from build123d import *

# Parameters (mm, degrees)
CROQUIS1_W              = 51
CROQUIS1_H              = 39
CROQUIS1_W_2            = 47
CROQUIS1_H_2            = 35
SALIENTE_EXTRUIR1_DEPTH = 36
CROQUIS2_W              = 51
CROQUIS2_H              = 39
SALIENTE_EXTRUIR2_DEPTH = 2
CROQUIS3_W              = 5
CROQUIS3_H              = 39
SALIENTE_EXTRUIR3_DEPTH = 2
CROQUIS4_W              = 51
CROQUIS4_H              = 2
CORTAR_EXTRUIR1_DEPTH   = 50.744346412
CROQUIS5_W              = 3
CROQUIS5_H              = 2
SALIENTE_EXTRUIR4_DEPTH = 35
REDONDEO1_R             = 2
CHAFL_N1_SIZE           = 1
CROQUIS6_W              = 35
CROQUIS6_H              = 10
CORTAR_EXTRUIR2_DEPTH   = 66.40068807


with BuildPart() as part:
    # Croquis1 → Saliente-Extruir1 (new body)
    with BuildSketch(Plane(origin=(0, 0, 0), x_dir=(1, 0, 0), z_dir=(0, 1, 0))):
        Rectangle(CROQUIS1_W, CROQUIS1_H)
        Rectangle(CROQUIS1_W_2, CROQUIS1_H_2, mode=Mode.SUBTRACT)
    extrude(amount=SALIENTE_EXTRUIR1_DEPTH)

    # Croquis2 → Saliente-Extruir2 (add)
    with BuildSketch(Plane.XZ):
        Rectangle(CROQUIS2_W, CROQUIS2_H)
    extrude(amount=SALIENTE_EXTRUIR2_DEPTH)

    # Croquis3 → Saliente-Extruir3 (add)
    with BuildSketch(Plane(origin=(0, 36, 0), x_dir=(1, 0, 0), z_dir=(0, 1, 0))):
        with Locations((-23, 0)):
            Rectangle(CROQUIS3_W, CROQUIS3_H)
        with Locations((23, 0)):
            Rectangle(CROQUIS3_W, CROQUIS3_H)
    extrude(amount=-SALIENTE_EXTRUIR3_DEPTH)

    # Croquis4 → Cortar-Extruir1 (cut, through all)
    with BuildSketch(Plane(origin=(0, 36, 0), x_dir=(1, 0, 0), z_dir=(0, 1, 0))):
        with Locations((0, -18.5)):
            Rectangle(CROQUIS4_W, CROQUIS4_H)
    extrude(amount=-CORTAR_EXTRUIR1_DEPTH, mode=Mode.SUBTRACT)

    # Croquis5 → Saliente-Extruir4 (add)
    with BuildSketch(Plane.XY.offset(17.5)):
        with Locations((-22, 30)):
            Rectangle(CROQUIS5_W, CROQUIS5_H)
        with Locations((22, 30)):
            Rectangle(CROQUIS5_W, CROQUIS5_H)
    extrude(amount=-SALIENTE_EXTRUIR4_DEPTH)

    # Redondeo1
    redondeo1_edges = [part.edges().sort_by_distance(p)[0] for p in [
        (-25.5, 36, -1),
        (0, 36, -19.5),
        (25.5, 36, -1),
    ]]
    fillet(redondeo1_edges, radius=REDONDEO1_R - 0.0001)  # a hair under: the kernel refuses the full size

    # Chaflán1
    chafl_n1_edges = [part.edges().sort_by_distance(p)[0] for p in [
        (-22, 31, 17.5),
        (22, 31, 17.5),
        (-22, 34, 17.5),
        (22, 34, 17.5),
    ]]
    chamfer(chafl_n1_edges, length=CHAFL_N1_SIZE)

    # Croquis6 → Cortar-Extruir2 (cut, through all)
    with BuildSketch(Plane(origin=(25.5, 0, 0), x_dir=(0, 0, -1), z_dir=(1, 0, 0))):
        with Locations((0, 3)):
            Rectangle(CROQUIS6_W, CROQUIS6_H)
    extrude(amount=-CORTAR_EXTRUIR2_DEPTH, mode=Mode.SUBTRACT)


solid = part.part
The model under review builds one solid part; all positions refer to its coordinate system, in mm. A direction names the side the tool comes from. Give positions to 0.01 mm unless a question says otherwise; leave off trailing zeros. Write each loop counter-clockwise with the first axis right and the second up, starting at its lowest first coordinate (ties: lowest second). Pieces come first, ordered by that corner, then holes. Notation, with made-up numbers: M -26.75,80 L 6.25,80 A27 ccw 6.25,99 Z; hole C 58,52.25 d5. An arc over 180 degrees is marked long. One line per question, with ' | ' between items. Start each with the question number.
Item 1: For faces 4 (the flat face through (-22, 34, -1)), 5 (the flat face through (-22, 29, 0)), 6 (the flat face through (-20.5, 35, 0)), 7 (the flat face through (-24, 8, 0)), list the 3-axis set-ups (+Z, -Z, +X, -X, +Y, -Y) from which the entire face can be reached by the end or side of a thin tool; tool diameter is ignored.
Item 2: We need section B-B on y = 15.5. Write out the cut boundary in (x, z), plus the area to 3 significant figures.
Item 3: For pin 1 (11.5 mm diameter, centred on x = 12.5, y = 12.5, fed in from +Z); pin 2 (2.5 mm diameter, centred on x = 21.5, z = 1, fed in from -Y); pin 3 (1.6 mm diameter, centred on y = 35, z = -1.5, fed in from +X), all flat-tipped, find the tip position at first contact; note any pin that passes through.
Item 4: We need section A-A on z = 7.5. Write out the cut boundary in (x, y).
Item 5: Draft analysis for pull direction Y (two halves, no side actions). For faces 1 (the flat face through (-25.5, 20, -1)), 2 (the flat face through (23.5, 32, 0)), 3 (the flat face through (22, 29, 0)), state which applies: released by +Y, released by -Y, zero draft, split by the parting line, or undercut.
Item 6: Wall thickness on line 1 (X direction, y = 24.5, z = 10); line 2 (Y direction, x = 21, z = 0); line 3 (Z direction, x = -7.5, y = 14.5): over which ranges is each line inside the solid? List them lowest first. Write a range as from..to.
Results found:
1) face 4: +Z | face 5: +Z, -Y | face 6: +Z, +Y, -Y | face 7: +Z, +X, -X, -Y
2) outline: M -25.5,-19.5 L 25.5,-19.5 L 25.5,17.5 L 23.5,17.5 L 23.5,-17.5 L -23.5,-17.5 L -23.5,17.5 L -25.5,17.5 Z | area: 242 mm2
3) pin 1: stops at z = -17.5 | pin 2: stops at y = 29 | pin 3: stops at x = 25.49
4) outline: M -25.5,8 L -23.5,8 L -23.5,29 L -20.5,29 L -20.5,31 L -23.5,31 L -23.5,34 L -20.5,34 L -20.5,36 L -23.5,36 A2 ccw -25.5,34 Z; M 20.5,29 L 23.5,29 L 23.5,8 L 25.5,8 L 25.5,34 A2 ccw 23.5,36 L 20.5,36 L 20.5,34 L 23.5,34 L 23.5,31 L 20.5,31 Z
5) face 1: zero draft | face 2: undercut | face 3: released by -Y
6) line 1: x = -25.5..-23.5, 23.5..25.5 | line 2: y = 29..31, 34..36 | line 3: z = -19.5..-17.5
